The listing builds one solid part. Answer for the finished solid, in the listing's coordinates (mm). Face numbers are marked on the shaded views. A direction names the side the tool comes from. Give positions to 0.01 mm unless a question says otherwise; leave off trailing zeros. Loops run counter-clockwise (first coordinate to the right, second up) from the corner with the lowest first, then second, coordinate; pieces in that order, holes last.
Item 1: The mould has two halves that part along Y. Classify the marked faces 1, 2 and 3: pulls with the +Y half, pulls with the -Y half, needs draft (parallel to the pull), parting line crosses it, or undercut.
Item 2: Section A-A, the plane z = 11.5 is taken. Give the vertices of the cut face in (x, y), and give its area (3 significant figures).
Item 3: Section B-B, the plane y = -5.5 is taken. Give the vertices of the cut face in (x, z).
Item 4: Consider line 1 along Y through (x, z) = (-23.9, 11.25); line 2 along Y through (x, z) = (0, 2.3); line 3 along Y through (x, z) = (10, 9.5). Determine where each line is inside the solid, lowest interval first.
Item 5: Each of these flat-tipped pins is pushed along its axis until it touches: pin 1 Ø1.4 at (x, y) = (-25, -23) entering from +Z; pin 2 Ø16 at (x, y) = (-1, -4) entering from +Z. Where does it stop, or does it pass through?
Item 6: A tool of negligible diameter and unlimited length cuts with its end or side. For the marked faces 4 and 5, from which of +Z, -Z, +X, -X, +Y, -Y can it reach the whole face along a straight path? Write none if from no direction.
Item 7: Section C-C, the plane x = -8.5 is taken. Give the vertices of the cut face in (y, z).
from build123d import *

# Parameters (mm, degrees)
SKICA1_W                 = 55.6
SKICA1_H                 = 55.6
P_IDAT_VYSUNUT_M2_DEPTH  = 3
SKICA5_W                 = 5
SKICA5_H                 = 25.3
ODEBRAT_VYSUNUT_M3_DEPTH = 1
SKICA14_W                = 53.6
SKICA14_H                = 1.5
P_IDAT_VYSUNUT_M9_DEPTH  = 9.5
SKICA17_R                = 2
ODEBRAT_VYSUNUT_M8_DEPTH = 4
SKICA19_W                = 6.8
SKICA19_H                = 6.8
P_IDAT_VYSUNUT_M10_DEPTH = 12.5
SKICA20_R                = 2.4
ODEBRAT_VYSUNUT_M9_DEPTH = 1.7
ZAOBLIT1_R               = 2.5
ZAOBLIT2_R               = 15
ZAOBLIT3_R               = 20


with BuildPart() as part:
    # Skica1 → Přidat vysunutím2 (new body)
    with BuildSketch(Plane.XY):
        Rectangle(SKICA1_W, SKICA1_H)
    extrude(amount=P_IDAT_VYSUNUT_M2_DEPTH)

    # Skica5 → Odebrat vysunutím3 (cut)
    with BuildSketch(Plane(origin=(0, 0, 0), x_dir=(-1, 0, 0), z_dir=(0, 0, -1))):
        Polygon((-2.5, 2.5), (-27.8, 2.5), (-27.8, -2.5), (2.5, -2.5), (2.5, 2.5), align=None)
        with Locations((0, 15.15)):
            Rectangle(SKICA5_W, SKICA5_H)
    extrude(amount=-ODEBRAT_VYSUNUT_M3_DEPTH, mode=Mode.SUBTRACT)

    # Skica14 → Přidat vysunutím9 (add)
    with BuildSketch(Plane.XY.offset(3)):
        Polygon((27.8, 27.8), (-27.8, 27.8), (-27.8, -27.8), (-26.8, -27.8), (-26.8, -26.8), (-26.8, -26.3), (-26.8, 26.8), (26.8, 26.8), (26.8, -26.3), (26.8, -27.8), (27.8, -27.8), align=None)
        with Locations((0, -27.05)):
            Rectangle(SKICA14_W, SKICA14_H)
    extrude(amount=P_IDAT_VYSUNUT_M9_DEPTH)

    # Skica17 → Odebrat vysunutím8 (cut)
    with BuildSketch(Plane(origin=(0, 0, 1), x_dir=(-1, 0, 0), z_dir=(0, 0, -1))):
        with Locations((-20.8, 0)):
            Circle(SKICA17_R)
        with Locations((0, 20.8)):
            Circle(SKICA17_R)
    extrude(amount=-ODEBRAT_VYSUNUT_M8_DEPTH, mode=Mode.SUBTRACT)

    # Skica19 → Přidat vysunutím10 (add)
    with BuildSketch(Plane(origin=(0, 0, 0), x_dir=(-1, 0, 0), z_dir=(0, 0, -1))):
        with Locations((-24.4, 24.4)):
            Rectangle(SKICA19_W, SKICA19_H)
        with Locations((24.4, 24.4)):
            Rectangle(SKICA19_W, SKICA19_H)
        with Locations((-24.4, -24.4)):
            Rectangle(SKICA19_W, SKICA19_H)
        with Locations((24.4, -24.4)):
            Rectangle(SKICA19_W, SKICA19_H)
    extrude(amount=-P_IDAT_VYSUNUT_M10_DEPTH)

    # Skica20 → Odebrat vysunutím9 (cut)
    with BuildSketch(Plane.XY.offset(12.5)):
        with Locations((-23.9, -23.9)):
            Circle(SKICA20_R)
        with Locations((-23.9, 23.9)):
            Circle(SKICA20_R)
        with Locations((23.900280565, 23.9)):
            Circle(SKICA20_R)
        with Locations((23.900280565, -23.9)):
            Circle(SKICA20_R)
    extrude(amount=-ODEBRAT_VYSUNUT_M9_DEPTH, mode=Mode.SUBTRACT)

    # Zaoblit1
    zaoblit1_edges = [part.edges().sort_by_distance(p)[0] for p in [
        (-21, 21, 7.75),
        (21, -21, 7.75),
        (-21, -21, 7.75),
        (21, 21, 7.75),
    ]]
    fillet(zaoblit1_edges, radius=ZAOBLIT1_R)

    # Zaoblit2
    zaoblit2_edges = [part.edges().sort_by_distance(p)[0] for p in [
        (2.5, 2.5, 0.5),
    ]]
    fillet(zaoblit2_edges, radius=ZAOBLIT2_R)

    # Zaoblit3
    zaoblit3_edges = [part.edges().sort_by_distance(p)[0] for p in [
        (-2.5, -2.5, 0.5),
    ]]
    fillet(zaoblit3_edges, radius=ZAOBLIT3_R)


solid = part.part
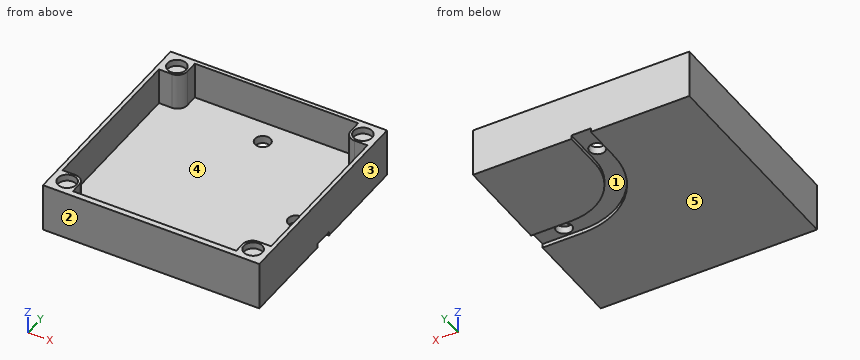
Worked answers:
1. face 1: undercut
1. face 2: pulls with the -Y half
1. face 3: needs draft
2. outline: (-27.8, -27.8) - (27.8, -27.8) - (27.8, 27.8) - (-27.8, 27.8) - close; hole (-26.8, -21) - (-23.5, -21) arc R2.5 cw to (-21, -23.5) - (-21, -26.3) - (21, -26.3) - (21, -23.5) arc R2.5 cw to (23.5, -21) - (26.8, -21) - (26.8, 21) - (23.5, 21) arc R2.5 cw to (21, 23.5) - (21, 26.8) - (-21, 26.8) - (-21, 23.5) arc R2.5 cw to (-23.5, 21) - (-26.8, 21) - close; hole circle Ø4.8 at (-23.9, -23.9); hole circle Ø4.8 at (-23.9, 23.9); hole circle Ø4.8 at (23.9, -23.9); hole circle Ø4.8 at (23.9, 23.9)
2. area: 296 mm2
3. outline: (-27.8, 0) - (27.8, 0) - (27.8, 12.5) - (26.8, 12.5) - (26.8, 3) - (-26.8, 3) - (-26.8, 12.5) - (-27.8, 12.5) - close
4. line 1: y = -27.8 to -26.3, -21.5 to -21, 21 to 21.5, 26.3 to 27.8
4. line 2: y = -27.8 to 18.8, 22.8 to 27.8
4. line 3: y = -27.8 to -26.3, 26.8 to 27.8
5. pin 1: stops at z = 10.8
5. pin 2: stops at z = 3
6. face 4: +Z
6. face 5: -Z, +X, -X, +Y, -Y
7. outline: (-27.8, 0) - (27.8, 0) - (27.8, 12.5) - (26.8, 12.5) - (26.8, 3) - (-26.3, 3) - (-26.3, 12.5) - (-27.8, 12.5) - close
